For this review, take the finished solid that the model builds, in its own axes (mm). A direction names the side the tool comes from. Give positions to 0.01 mm unless a question says otherwise; leave off trailing zeros. Write each loop counter-clockwise with the first axis right and the second up, starting at its lowest first coordinate (ties: lowest second). Pieces come first, ordered by that corner, then holes. Notation, with made-up numbers: M 23,-26.75 L 62,-26.75 A20 cw 62,-13.75 Z; hole C 16,18.25 d9. An arc over 180 degrees is marked long. One line per item, written item: value. Start each with the question number.
Item 1: Tool access review of faces 1 (the face through (-13.22, -165.34, -59.55)), 2 (the face through (-48.408, -9.663, -37.118)): name each direction out of +Z, -Z, +X, -X, +Y, -Y from which nothing blocks a thin tool from reaching the whole face with its end or side.
Item 2: Clearance check with flat-ended pins moving along their axes: pin 1 Ø5 at (x, y) = (-25.5, -135.5) entering from -Z; pin 2 Ø8 at (y, z) = (-120, 45) entering from +X; pin 3 Ø10 at (x, y) = (-49, -119) entering from +Z. State where each tip first meets the part, or that it passes through.
Item 3: Consider section B-B, the plane z = 0. Write out the cut boundary in (x, y), and give its area (3 significant figures).
Item 4: Consider section C-C, the plane y = -26. Write out the cut boundary in (x, z).
Item 5: Consider section A-A, the plane x = 0. Write out the cut boundary in (y, z), and give its area (3 significant figures).
Item 6: To check wall thickness, follow probe 1 along Z at (x, y) = (0, -63.5); probe 2 along Z at (x, y) = (16, -64); probe 3 along X at (y, z) = (-44, -39.5). State the ranges of each line that lie inside material, in increasing order.
Item 7: Mouldability with a two-part tool opening along Z and no side actions: class faces 3 (the face through (-24, -155.8, 57)), 4 (the face through (-13.77, -86.54, -61.99)), 5 (the face through (-7.601, -86.317, 57.893)), 6 (the face through (-12.69, -2.87, -57.13)) as released by +Z, released by -Z, zero draft, split by the parting line, or undercut.
```python
from build123d import *

# Parameters (mm, degrees)
F0_R     = 63.5
F0_R_2   = 58.39
F1_DEPTH = 175
F2_R     = 63.5
F2_R_2   = 61
F3_DEPTH = 19.2
F4_R     = 63.5
F4_R_2   = 61
F5_DEPTH = 19.2


# Not quite as in the source:
# - a fillet or chamfer that OpenCascade refuses, or shapes differently, is made with other operations: its cross-section is extruded or revolved along the edge and cut away or added


with BuildPart() as f1:
    # F0 (on Front) → F1 (new body)
    with BuildSketch(Plane.XZ):
        Circle(F0_R)
        Circle(F0_R_2, mode=Mode.SUBTRACT)
    extrude(amount=F1_DEPTH)

    # F2 (on Front) → F3 (cut)
    with BuildSketch(Plane.XZ):
        Circle(F2_R)
        Circle(F2_R_2, mode=Mode.SUBTRACT)
    extrude(amount=F3_DEPTH, mode=Mode.SUBTRACT)

    # F4 (on face) → F5 (cut)
    with BuildSketch(Plane.XZ.offset(175)):
        Circle(F4_R)
        Circle(F4_R_2, mode=Mode.SUBTRACT)
    extrude(amount=-F5_DEPTH, mode=Mode.SUBTRACT)

    # F6: chamfer of 3 on 2 edges, made by hand

    # F6_s1 → F6_t2 (revolve, cut)
    with BuildSketch(Plane.XY):
        Polygon((61.39, -175), (58.39, -172), (58.39, -175), align=None)
    revolve(axis=Axis((0, -175, 0), (0, -1, 0)), mode=Mode.SUBTRACT)

    # F6_s3 → F6_t4 (revolve, cut)
    with BuildSketch(Plane.XY):
        Polygon((61.39, 0), (58.39, -3), (58.39, 0), align=None)
    revolve(axis=Axis((0, 0, 0), (0, -1, 0)), mode=Mode.SUBTRACT)


solid = f1.part
```
Model answer:
1. face 1: -Y
1. face 2: +Y
2. pin 1: stops at z = -59.19
2. pin 2: stops at x = 48.49
2. pin 3: stops at z = 45.78
3. outline: M -63.5,-155.8 L -61,-155.8 L -61,-174.61 L -58.39,-172 L -58.39,-3 L -61,-0.39 L -61,-19.2 L -63.5,-19.2 Z; M 58.39,-172 L 61,-174.61 L 61,-155.8 L 63.5,-155.8 L 63.5,-19.2 L 61,-19.2 L 61,-0.39 L 58.39,-3 Z
3. area: 1,580 mm2
4. outline: C 0,0 d127; hole C 0,0 d116.78
5. outline: M -174.61,-61 L -155.8,-61 L -155.8,-63.5 L -19.2,-63.5 L -19.2,-61 L -0.39,-61 L -3,-58.39 L -172,-58.39 Z; M -174.61,61 L -172,58.39 L -3,58.39 L -0.39,61 L -19.2,61 L -19.2,63.5 L -155.8,63.5 L -155.8,61 Z
5. area: 1,580 mm2
6. probe 1: z = -63.5 to -58.39, 58.39 to 63.5
6. probe 2: z = -61.45 to -56.16, 56.16 to 61.45
6. probe 3: x = -49.72 to -43, 43 to 49.72
7. face 3: zero draft
7. face 4: split by the parting line
7. face 5: undercut
7. face 6: undercut
